```python
from build123d import *

# Parameters (mm, degrees)
F0_W      = 50.8
F0_H      = 69.85
F1_DEPTH  = 146.05
F3_DEPTH  = 69.851
F4_R      = 13.843
F5_DEPTH  = 7.112
F6_SIZE   = 22.225
F7_W      = 3.175
F7_H      = 146.05
F8_DEPTH  = 9.525
F10_DEPTH = 7.112


with BuildPart() as f1:
    # F0 (on Top) → F1 (new body)
    with BuildSketch(Plane.XY):
        with Locations((25.4, 34.925)):
            Rectangle(F0_W, F0_H)
    extrude(amount=F1_DEPTH)

    # F2 (on face) → F3 (cut, through all)
    with BuildSketch(Plane.XZ):
        Polygon((50.8, 146.05), (0, 146.05), (50.8, 93.7700346112), align=None)
    extrude(amount=-F3_DEPTH, mode=Mode.SUBTRACT)

    # F4 (on face) → F5 (cut)
    with BuildSketch(Plane(origin=(72.9948999902, 0, 70.9285266723), x_dir=(0, 1, 0), z_dir=(0.7171851159, 0, 0.6968827086))):
        with Locations((34.925, 68.2968588571)):
            Circle(F4_R)
    extrude(amount=-F5_DEPTH, mode=Mode.SUBTRACT)

    # F6
    f6_edges = [f1.edges().sort_by_distance(p)[0] for p in [
        (50.8, 0, 46.885017),
        (50.8, 69.85, 46.885017),
        (0, 69.85, 73.025),
        (0, 0, 73.025),
    ]]
    chamfer(f6_edges, length=F6_SIZE)

    # F7 (on face) → F8 (cut)
    with BuildSketch(Plane(origin=(0, 0, 0), x_dir=(0, -1, 0), z_dir=(-1, 0, 0))):
        with Locations((-34.925, 73.025)):
            Rectangle(F7_W, F7_H)
    extrude(amount=-F8_DEPTH, mode=Mode.SUBTRACT)

    # F9 (on face) → F10 (cut)
    with BuildSketch(Plane(origin=(72.9948999902, 0, 70.9285266723), x_dir=(0, 1, 0), z_dir=(0.7171851159, 0, 0.6968827086))):
        with BuildLine():
            Line((36.5125, 91.0768759299), (33.3375, 91.0768759299))
            Line((33.3375, 91.0768759299), (33.3375, 82.048531219))
            ThreePointArc((33.3375, 82.048531219), (34.925, 82.1398588571), (36.5125, 82.048531219))
            Line((36.5125, 82.048531219), (36.5125, 91.0768759299))
        make_face()
    extrude(amount=-F10_DEPTH, mode=Mode.SUBTRACT)


solid = f1.part
```
Geometry check sheet. Reference: the model listing, model coordinates, mm. A direction names the side the tool comes from. Coordinates: 2 decimals unless noted, no trailing zeros. Order: outer loops, then holes, each group sorted by start corner. A loop starts at its lowest first (then second) coordinate and runs counter-clockwise, first axis right, second up. Notation, with made-up numbers: (41, 25) - (74, 25) arc R15 cw to (74, 46) - close; hole circle Ø2 at (-31.75, 61). An arc over 180 degrees is marked (long way). Answer in a Markdown table with one row per item. Add a question column.
1. Material ranges on L1, parallel to Y at x = 2, z = 65.5 (1 decimal); L2, parallel to Z at x = 20, y = 19.5; L3, parallel to Y at x = 38, z = 30 (3 decimals), recorded low to high. Write a range as [from, to].
2. Section check A-A (x = 8). Enter the section's corners in (y, z) (1 decimal), plus the area to 3 significant figures.
3. Gauge pin test, flat ends, axial feed: pin 1 Ø8 at (x, z) = (5, 102.5) entering from -Y (3 decimals); pin 2 Ø6 at (x, z) = (35, 67.5) entering from +Y (3 decimals); pin 3 Ø3.5 at (y, z) = (35, 37) entering from -X; pin 4 Ø12.5 at (x, z) = (9, 84) entering from +Y (3 decimals). Record the tip position at first contact, or that the pin passes through.
4. Access from +Z, -Z, +X, -X, +Y, -Y to the whole of each face (thin tool, end or side, straight path). Record for faces 1 (the face through (9.525, 35, 64)), 2 (the face through (11.268, 10.957, 72.003)), 3 (the face through (19.593, 34.731, 115.681)).
5. Section check C-C (y = 40). Enter the section's corners in (x, z), plus the area to 3 significant figures.
6. Draft check along Y on faces 4 (the face through (32.524, 34.339, 107.548)), 5 (the face through (0, 42, 72)), 6 (the face through (39.843, 58.582, 57.505)). Enter one of: +Y half, -Y half, draft (parallel to the pull), parting line (faces both ways), or undercut.
Data:
| question | item | result |
|---|---|---|
| 1 | L1 | y = [20.2, 33.3], [36.5, 49.6] |
| 1 | L2 | z = [0, 125.47] |
| 1 | L3 | y = [9.425, 60.425] |
| 2 | outline | (14.2, 0) - (33.3, 0) - (33.3, 137.8) - (14.2, 137.8) - close; (36.5, 0) - (55.6, 0) - (55.6, 137.8) - (36.5, 137.8) - close |
| 2 | area | 5,270 mm² |
| 3 | pin 1 | stops at y = 13.225 |
| 3 | pin 2 | stops at y = 66.425 |
| 3 | pin 3 | stops at x = 0 |
| 3 | pin 4 | stops at y = 62.875 |
| 4 | face 1 | +Z, -Z, -X |
| 4 | face 2 | +Z, -Z, -X, -Y |
| 4 | face 3 | none |
| 5 | outline | (0, 0) - (50.8, 0) - (50.8, 93.77) - (34.38, 110.67) - (29.27, 105.72) - (11.32, 124.19) - (16.42, 129.15) - (0, 146.05) - close |
| 5 | area | 5,910 mm² |
| 6 | face 4 | undercut |
| 6 | face 5 | draft |
| 6 | face 6 | +Y half |
